Read the model definition and answer for the solid it produces. Units are mm, in the model's axes. Round coordinates to 2 decimals unless told otherwise and drop trailing zeros. Order: outer loops, then holes, each group sorted by start corner. A loop starts at its lowest first (then second) coordinate and runs counter-clockwise, first axis right, second up. Notation, with made-up numbers: M 78.25,6.25 L 110.25,6.25 A32 ccw 110.25,32.25 Z; hole C 5.25,5 d7. An arc over 180 degrees is marked long. Answer as CSV lines item,"result".
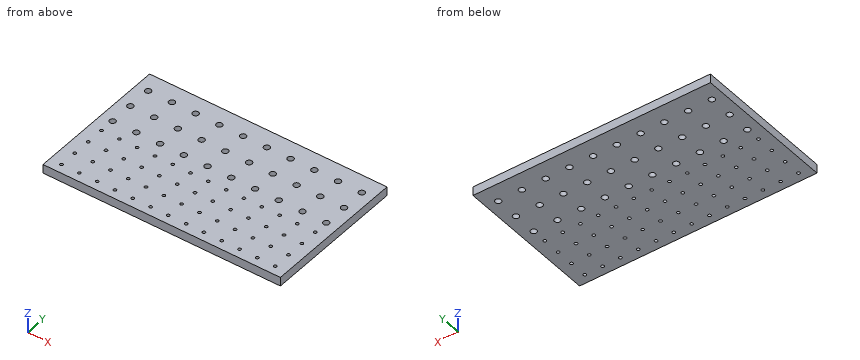
```python
from build123d import *

# Parameters (mm, degrees)
F0_W     = 508
F0_H     = 304.8
F0_R     = 3.2385
F0_R_2   = 6.4135
F1_DEPTH = 19.05


with BuildPart() as f1:
    # F0 (on Top) → F1 (new body)
    with BuildSketch(Plane.XY):
        Rectangle(F0_W, F0_H)
        with Locations((-228.6, -133.35)):
            Circle(F0_R, mode=Mode.SUBTRACT)
        with Locations((-190.5, -133.35)):
            Circle(F0_R, mode=Mode.SUBTRACT)
        with Locations((-152.4, -133.35)):
            Circle(F0_R, mode=Mode.SUBTRACT)
        with Locations((-228.6, -95.25)):
            Circle(F0_R, mode=Mode.SUBTRACT)
        with Locations((-190.5, -95.25)):
            Circle(F0_R, mode=Mode.SUBTRACT)
        with Locations((-152.4, -95.25)):
            Circle(F0_R, mode=Mode.SUBTRACT)
        with Locations((-114.3, -133.35)):
            Circle(F0_R, mode=Mode.SUBTRACT)
        with Locations((-76.2, -133.35)):
            Circle(F0_R, mode=Mode.SUBTRACT)
        with Locations((-38.1, -133.35)):
            Circle(F0_R, mode=Mode.SUBTRACT)
        with Locations((-114.3, -95.25)):
            Circle(F0_R, mode=Mode.SUBTRACT)
        with Locations((-76.2, -95.25)):
            Circle(F0_R, mode=Mode.SUBTRACT)
        with Locations((-38.1, -95.25)):
            Circle(F0_R, mode=Mode.SUBTRACT)
        with Locations((-228.6, -57.15)):
            Circle(F0_R, mode=Mode.SUBTRACT)
        with Locations((-190.5, -57.15)):
            Circle(F0_R, mode=Mode.SUBTRACT)
        with Locations((-152.4, -57.15)):
            Circle(F0_R, mode=Mode.SUBTRACT)
        with Locations((-228.6, -19.05)):
            Circle(F0_R, mode=Mode.SUBTRACT)
        with Locations((-190.5, -19.05)):
            Circle(F0_R, mode=Mode.SUBTRACT)
        with Locations((-152.4, -19.05)):
            Circle(F0_R, mode=Mode.SUBTRACT)
        with Locations((-114.3, -57.15)):
            Circle(F0_R, mode=Mode.SUBTRACT)
        with Locations((-76.2, -57.15)):
            Circle(F0_R, mode=Mode.SUBTRACT)
        with Locations((-38.1, -57.15)):
            Circle(F0_R, mode=Mode.SUBTRACT)
        with Locations((-114.3, -19.05)):
            Circle(F0_R, mode=Mode.SUBTRACT)
        with Locations((-76.2, -19.05)):
            Circle(F0_R, mode=Mode.SUBTRACT)
        with Locations((-38.1, -19.05)):
            Circle(F0_R, mode=Mode.SUBTRACT)
        with Locations((0, -133.35)):
            Circle(F0_R, mode=Mode.SUBTRACT)
        with Locations((38.1, -133.35)):
            Circle(F0_R, mode=Mode.SUBTRACT)
        with Locations((76.2, -133.35)):
            Circle(F0_R, mode=Mode.SUBTRACT)
        with Locations((114.3, -133.35)):
            Circle(F0_R, mode=Mode.SUBTRACT)
        with Locations((0, -95.25)):
            Circle(F0_R, mode=Mode.SUBTRACT)
        with Locations((38.1, -95.25)):
            Circle(F0_R, mode=Mode.SUBTRACT)
        with Locations((76.2, -95.25)):
            Circle(F0_R, mode=Mode.SUBTRACT)
        with Locations((114.3, -95.25)):
            Circle(F0_R, mode=Mode.SUBTRACT)
        with Locations((152.4, -133.35)):
            Circle(F0_R, mode=Mode.SUBTRACT)
        with Locations((190.5, -133.35)):
            Circle(F0_R, mode=Mode.SUBTRACT)
        with Locations((228.6, -133.35)):
            Circle(F0_R, mode=Mode.SUBTRACT)
        with Locations((152.4, -95.25)):
            Circle(F0_R, mode=Mode.SUBTRACT)
        with Locations((190.5, -95.25)):
            Circle(F0_R, mode=Mode.SUBTRACT)
        with Locations((228.6, -95.25)):
            Circle(F0_R, mode=Mode.SUBTRACT)
        with Locations((0, -57.15)):
            Circle(F0_R, mode=Mode.SUBTRACT)
        with Locations((38.1, -57.15)):
            Circle(F0_R, mode=Mode.SUBTRACT)
        with Locations((76.2, -57.15)):
            Circle(F0_R, mode=Mode.SUBTRACT)
        with Locations((114.3, -57.15)):
            Circle(F0_R, mode=Mode.SUBTRACT)
        with Locations((0, -19.05)):
            Circle(F0_R, mode=Mode.SUBTRACT)
        with Locations((38.1, -19.05)):
            Circle(F0_R, mode=Mode.SUBTRACT)
        with Locations((76.2, -19.05)):
            Circle(F0_R, mode=Mode.SUBTRACT)
        with Locations((114.3, -19.05)):
            Circle(F0_R, mode=Mode.SUBTRACT)
        with Locations((152.4, -57.15)):
            Circle(F0_R, mode=Mode.SUBTRACT)
        with Locations((190.5, -57.15)):
            Circle(F0_R, mode=Mode.SUBTRACT)
        with Locations((228.6, -57.15)):
            Circle(F0_R, mode=Mode.SUBTRACT)
        with Locations((152.4, -19.05)):
            Circle(F0_R, mode=Mode.SUBTRACT)
        with Locations((190.5, -19.05)):
            Circle(F0_R, mode=Mode.SUBTRACT)
        with Locations((228.6, -19.05)):
            Circle(F0_R, mode=Mode.SUBTRACT)
        with Locations((-228.6, 12.7)):
            Circle(F0_R_2, mode=Mode.SUBTRACT)
        with Locations((-177.8, 12.7)):
            Circle(F0_R_2, mode=Mode.SUBTRACT)
        with Locations((-228.6, 63.5)):
            Circle(F0_R_2, mode=Mode.SUBTRACT)
        with Locations((-177.8, 63.5)):
            Circle(F0_R_2, mode=Mode.SUBTRACT)
        with Locations((-127, 12.7)):
            Circle(F0_R_2, mode=Mode.SUBTRACT)
        with Locations((-76.2, 12.7)):
            Circle(F0_R_2, mode=Mode.SUBTRACT)
        with Locations((-25.4, 12.7)):
            Circle(F0_R_2, mode=Mode.SUBTRACT)
        with Locations((-127, 63.5)):
            Circle(F0_R_2, mode=Mode.SUBTRACT)
        with Locations((-76.2, 63.5)):
            Circle(F0_R_2, mode=Mode.SUBTRACT)
        with Locations((-25.4, 63.5)):
            Circle(F0_R_2, mode=Mode.SUBTRACT)
        with Locations((-228.6, 114.3)):
            Circle(F0_R_2, mode=Mode.SUBTRACT)
        with Locations((-177.8, 114.3)):
            Circle(F0_R_2, mode=Mode.SUBTRACT)
        with Locations((-127, 114.3)):
            Circle(F0_R_2, mode=Mode.SUBTRACT)
        with Locations((-76.2, 114.3)):
            Circle(F0_R_2, mode=Mode.SUBTRACT)
        with Locations((-25.4, 114.3)):
            Circle(F0_R_2, mode=Mode.SUBTRACT)
        with Locations((25.4, 12.7)):
            Circle(F0_R_2, mode=Mode.SUBTRACT)
        with Locations((76.2, 12.7)):
            Circle(F0_R_2, mode=Mode.SUBTRACT)
        with Locations((25.4, 63.5)):
            Circle(F0_R_2, mode=Mode.SUBTRACT)
        with Locations((76.2, 63.5)):
            Circle(F0_R_2, mode=Mode.SUBTRACT)
        with Locations((127, 12.7)):
            Circle(F0_R_2, mode=Mode.SUBTRACT)
        with Locations((177.8, 12.7)):
            Circle(F0_R_2, mode=Mode.SUBTRACT)
        with Locations((228.6, 12.7)):
            Circle(F0_R_2, mode=Mode.SUBTRACT)
        with Locations((127, 63.5)):
            Circle(F0_R_2, mode=Mode.SUBTRACT)
        with Locations((177.8, 63.5)):
            Circle(F0_R_2, mode=Mode.SUBTRACT)
        with Locations((228.6, 63.5)):
            Circle(F0_R_2, mode=Mode.SUBTRACT)
        with Locations((25.4, 114.3)):
            Circle(F0_R_2, mode=Mode.SUBTRACT)
        with Locations((76.2, 114.3)):
            Circle(F0_R_2, mode=Mode.SUBTRACT)
        with Locations((127, 114.3)):
            Circle(F0_R_2, mode=Mode.SUBTRACT)
        with Locations((177.8, 114.3)):
            Circle(F0_R_2, mode=Mode.SUBTRACT)
        with Locations((228.6, 114.3)):
            Circle(F0_R_2, mode=Mode.SUBTRACT)
    extrude(amount=F1_DEPTH)


solid = f1.part
```
Item 1: Find the intervals of material crossed by probe 1 along Y at (x, z) = (114.3, 8.25); probe 2 along Y at (x, z) = (177.8, 5), in increasing order. Write a range as [from, to].
Ans:
probe 1,"[-152.4, -136.59], [-130.11, -98.49], [-92.01, -60.39], [-53.91, -22.29], [-15.81, 152.4]"
probe 2,"[-152.4, 6.29], [19.11, 57.09], [69.91, 107.89], [120.71, 152.4]"
Item 2: A cutting plane is placed at B-B, the plane y = 114.3. Give the number of separate pieces and of enclosed holes in the cut face, and give its area (3 significant figures).
Ans:
separate pieces,"11"
enclosed holes,"0"
area,"7,230 mm2"
Item 3: A cutting plane is placed at A-A, the plane x = -127. Determine the outline of the cut face in (y, z), and give its area (3 significant figures).
Ans:
outline,"M -152.4,0 L 6.29,0 L 6.29,19.05 L -152.4,19.05 Z; M 19.11,0 L 57.09,0 L 57.09,19.05 L 19.11,19.05 Z; M 69.91,0 L 107.89,0 L 107.89,19.05 L 69.91,19.05 Z; M 120.71,0 L 152.4,0 L 152.4,19.05 L 120.71,19.05 Z"
area,"5,070 mm2"
